```python
from build123d import *

# Parameters (mm, degrees)
F0_R     = 12
F1_DEPTH = 23.5


with BuildPart() as f1:
    # F0 (on Top) → F1 (new body, symmetric)
    with BuildSketch(Plane.XY):
        with BuildLine():
            ThreePointArc((10.8902694237, -6.2875000501), (12.1465172581, -3.2546495201), (12.575, 0))
            ThreePointArc((12.575, 0), (8.891867784, 8.8918677628), (2.99e-08, 12.575))
            ThreePointArc((2.99e-08, 12.575), (-10.8902693743, 6.2875001356), (-10.8902695943, -6.2874997546))
            ThreePointArc((-10.8902695943, -6.2874997546), (-1.706e-07, -12.575), (10.8902694237, -6.2875000501))
        make_face()
        Circle(F0_R, mode=Mode.SUBTRACT)
    extrude(amount=F1_DEPTH, both=True)


solid = f1.part
```
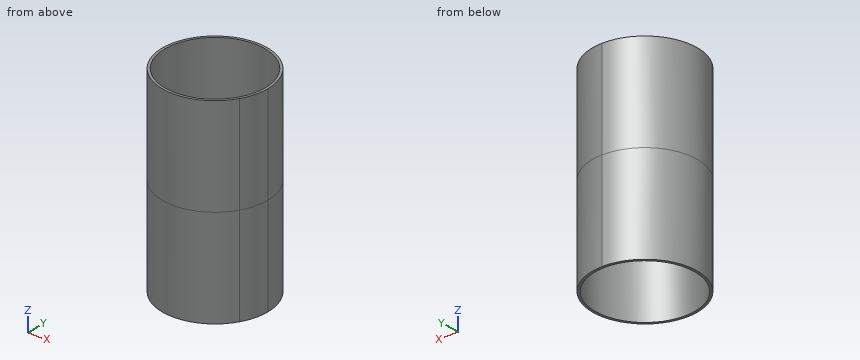
Check sheet for the modelled part. Datum: model origin and axes. Units: mm. Coordinates: 2 decimals unless noted, no trailing zeros. Loops run counter-clockwise (first coordinate to the right, second up) from the corner with the lowest first, then second, coordinate; pieces in that order, holes last.
1) Gauge pin test, flat ends, axial feed: pin 1 (3 mm diameter, centred on x = 9, z = 0, fed in from +Y); pin 2 (5 mm diameter, centred on y = -5.5, z = -14, fed in from +X); pin 3 (8 mm diameter, centred on x = 5.5, y = 3, fed in from +Z); pin 4 (1 mm diameter, centred on y = 4.5, z = 12, fed in from +X). Record the tip position at first contact, or that the pin passes through.
2) Material ranges on probe 1 along X at (y, z) = (0.5, 0.5); probe 2 along X at (y, z) = (6.75, -15); probe 3 along Y at (x, z) = (-0.75, 12), recorded low to high.
3) Sectioned sample at B-B (x = -8.25). Record the boundary of the cut face in (y, z), and give its area (3 significant figures).
4) Sectioned sample at C-C (y = -5.75). Record the boundary of the cut face in (x, z), and give its area (3 significant figures).
Check sheet entries:
1. pin 1: stops at y = 10.09
1. pin 2: stops at x = 12.21
1. pin 3: passes through
1. pin 4: stops at x = 11.92
2. probe 1: x = -12.57 to -11.99, 11.99 to 12.57
2. probe 2: x = -10.61 to -9.92, 9.92 to 10.61
2. probe 3: y = -12.55 to -11.98, 11.98 to 12.55
3. outline: (-9.49, -23.5) - (-8.71, -23.5) - (-8.71, 23.5) - (-9.49, 23.5) - close; (8.71, -23.5) - (9.49, -23.5) - (9.49, 23.5) - (8.71, 23.5) - close
3. area: 73.0 mm2
4. outline: (-11.18, -23.5) - (-10.53, -23.5) - (-10.53, 23.5) - (-11.18, 23.5) - close; (10.53, -23.5) - (11.18, -23.5) - (11.18, 23.5) - (10.53, 23.5) - close
4. area: 61.2 mm2
